Autodesk Inventor part; units mm, degrees
ref_plane "YZ Plane" through (0, 0, 0) normal (1, 0, 0) x (0, 1, 0)
ref_plane "XZ Plane" through (0, 0, 0) normal (0, 1, 0) x (-1, 0, 0)
ref_plane "XY Plane" through (0, 0, 0) normal (0, 0, 1) x (1, 0, 0)
sketch "Sketch1" plane through (0, 0, 0) normal (0, 1, 0) x (-1, 0, 0)
  line L0 (0.85, 10.55) -> (-0.85, 10.55)
  line L1 (-0.85, 10.55) -> (-0.85, -10.55)
  line L2 (-0.85, -10.55) -> (0.85, -10.55)
  line L3 (0.85, -10.55) -> (0.85, 10.55)
  line L4 (0.85, 10.55) -> (-0.85, -10.55) construction
  line L5 (-0.85, 10.55) -> (0.85, -10.55) construction
  line L6 (2.35, 12.05) -> (-2.35, 12.05)
  line L7 (-2.35, 12.05) -> (-2.35, -12.05)
  line L8 (-2.35, -12.05) -> (2.35, -12.05)
  line L9 (2.35, -12.05) -> (2.35, 12.05)
  point P0 (0, 0)
  dimension "d0" = 1.7
  dimension "d1" = 21.1
  dimension "d2" = 1.5
extrude "Extrusion1" add sketch "Sketch1" along normal blind 1.5
sketch "Sketch2" plane through (0, 0, 0) normal (0, -1, 0) x (1, 0, 0)
  line L0 (4.95, 12.05) -> (-6.05, 12.05)
  line L1 (-6.05, 12.05) -> (-6.05, -12.05)
  line L2 (-6.05, -12.05) -> (4.95, -12.05)
  line L3 (4.95, -12.05) -> (4.95, 12.05)
  line L4 (-2.35, 12.05) -> (2.35, 12.05)
  line L5 (-2.35, -12.05) -> (-2.35, 12.05)
  dimension "d5" = 11
  dimension "d6" = 3.7
extrude "Extrusion2" add sketch "Sketch2" along normal blind 2.4
sketch "Sketch3" plane through (0, 0, 0) normal (0, 1, 0) x (1, 0, 0)
  line L0 (-2.35, 12.05) -> (-2.35, -12.05)
  line L1 (-6.05, 12.05) -> (-2.35, 12.05)
  line L2 (-6.05, -12.05) -> (-6.05, 12.05)
  line L3 (-2.35, -12.05) -> (-6.05, -12.05)
  line L4 (2.35, -12.05) -> (2.35, 12.05)
  line L5 (4.95, -12.05) -> (2.35, -12.05)
  line L6 (4.95, 12.05) -> (4.95, -12.05)
  line L7 (2.35, 12.05) -> (4.95, 12.05)
  point P0 (0, 0)
extrude "Extrusion3" cut sketch "Sketch3" against normal blind 1.4
move faces "Move1" translate (0, 0, -1.5) faces at (0.7833, 0.5333, 12.05)
sketch "Sketch4" plane through (0, -2.4, 0) normal (0, -1, 0) x (1, 0, 0)
  line L0 (-0.85, -10.55) -> (0.85, -10.55)
  line L1 (-6.05, 10.55) -> (-6.05, -12.05)
  line L2 (2.35, -12.05) -> (4.95, -12.05)
  line L3 (-6.05, -10.55) -> (4.95, -10.55)
  line L4 (4.95, -10.55) -> (4.95, -12.05)
  line L5 (4.95, -12.05) -> (-6.05, -12.05)
  line L6 (-6.05, -12.05) -> (-6.05, -10.55)
  point P0 (0, 0)
extrude "Extrusion4" add sketch "Sketch4" along normal blind 1.8
move faces "Move2" translate (0, -1.4, 0) faces at (-0.2833, 0, 3.5167)
move faces "Move3" translate (0.5, 0, 0) faces at (-6.05, -1.7333, -4.0167)
move faces "Move4" translate (-0.5, 0, 0) faces at (4.95, -1.7333, -4.0167)
move faces "Move5" translate (0, 0, 1) faces at (-0.65, -2.0667, 10.55)
sketch "Sketch5" plane through (-5.55, -2.4, 11.55) normal (0, 0, 1) x (1, 0, 0)
  line L0 (4.7, 1) -> (4.7, 3.9)
  line L1 (3.2, 3.9) -> (4.7, 3.9)
  line L2 (3.2, 1) -> (3.2, 3.9)
  line L3 (3.2, 1) -> (0, 1)
  line L4 (0, 1) -> (0, 0)
  line L5 (10, 0) -> (0, 0)
  line L6 (10, 1) -> (10, 0)
  line L7 (10, 1) -> (7.9, 1)
  line L8 (7.9, 1) -> (7.9, 3.9)
  line L9 (6.4, 3.9) -> (7.9, 3.9)
  line L10 (6.4, 1) -> (6.4, 3.9)
  line L11 (6.4, 1) -> (4.7, 1)
  line L12 (4.7, 3.9) -> (6.4, 3.9)
  line L13 (4.7, 3.9) -> (6.4, 3.9)
  point P0 (5.55, 2.4)
extrude "Extrusion5" add sketch "Sketch5" along normal blind 1
move faces "Move6" translate (0, 0, -0.5) faces at (-0.2833, 0.5333, 11.55)
move faces "Move7" translate (0, 0.5, 0) faces at (-0.85, 0.5333, -3.35) (-0.2833, -1.4, -3.35)
sketch "Sketch6" plane through (2.35, -1.4, -12.05) normal (1, 0, 0) x (0, 0, -1)
  line L0 (-1.5, 2.9) -> (-23.1, 2.9)
  circle A0 centre (-3.41, 2.9) radius 0.75
  circle A1 centre (-5.95, 2.9) radius 0.75
  circle A2 centre (-8.49, 2.9) radius 0.75
  circle A3 centre (-11.03, 2.9) radius 0.75
  circle A4 centre (-13.57, 2.9) radius 0.75
  circle A5 centre (-16.11, 2.9) radius 0.75
  circle A6 centre (-18.65, 2.9) radius 0.75
  circle A7 centre (-21.19, 2.9) radius 0.75
  point P0 (-12.05, 1.4)
  dimension "d36" = 1.5
  dimension "d39" = 2.54
  dimension "d44" = 1.91
  dimension "d45" = 1.91
extrude "Extrusion6" cut sketch "Sketch6" against normal blind 2
equation "\"d44\" = d45"
properties part number "gyro_holder"
Could you check a few things on this model? Use its own coordinates, in mm. A direction names the side the tool comes from. Coordinates: 2 decimals unless noted, no trailing zeros. Order: outer loops, then holes, each group sorted by start corner. A loop starts at its lowest first (then second) coordinate and runs counter-clockwise, first axis right, second up. Notation, with made-up numbers: (-30, 30.5) - (27, 30.5) arc R17 cw to (27, 40.5) - close; hole circle Ø1 at (-29, 88.25). An arc over 180 degrees is marked (long way). Answer in a Markdown table with one row per item. Add a question column.
(1) On a 3-axis mill with a long thin cutter (end or side, diameter ignored), from which of +Z, -Z, +X, -X, +Y, -Y can I reach the whole of each face in a straight line? I mean faces 4 (the face through (1.61, 0.75, 6.62)), 5 (the face through (-0.85, 0, 0)), 6 (the face through (2.35, 0, 0)), 7 (the face through (2, 1.5, -2)). Say none if no direction works.
(2) If we mould it in two halves opening along X, with no side actions, what happens to faces 1 (the face through (-4, -1.4, 0)), 2 (the face through (-2.35, 0, 0)), 3 (the face through (0, 0, 11.05))? For each: released by +X, released by -X, zero draft, split by the parting line, or undercut.
(3) Will these pins go through, and if not, where does the flat tip stop? pin 1 (4 mm diameter, centred on x = -3.5, z = 3.5, fed in from -Y); pin 2 (1.9 mm diameter, centred on y = 0, z = -0.5, fed in from -X); pin 3 (2 mm diameter, centred on x = 0.5, y = -3, fed in from +Z); pin 4 (1.5 mm diameter, centred on y = 0.5, z = -1.5, fed in from +X).
(4) If we section it at B-B, the plane y = 0.25: Please give me the cut outline in (x, z), then the cut area to 3 significant figures.
(5) I need wall thicknesses on L1, parallel to X at y = -0.1, z = -2.5; L2, parallel to Y at x = -2.5, z = 0; L3, parallel to Y at x = 1, z = -5. Which ranges of each line are inside material? Lowest first, please.
(6) If we section it at A-A, the plane z = -8.64: Please give me the cut outline in (x, y).
(7) If we section it at D-D, the plane y = -2.7: Please give me the cut outline in (x, z), then the cut area to 3 significant figures.
(8) If we section it at C-C, the plane x = 2: Please give me the cut outline in (y, z).
Results are:
| question | item | result |
|---|---|---|
| 1 | face 4 | +X, +Y |
| 1 | face 5 | +Y |
| 1 | face 6 | +Z, -Z, +X, +Y |
| 1 | face 7 | +Z, -Z, +X, -X, +Y |
| 2 | face 1 | zero draft |
| 2 | face 2 | released by -X |
| 2 | face 3 | undercut |
| 3 | pin 1 | stops at y = -2.4 |
| 3 | pin 2 | stops at x = -2.35 |
| 3 | pin 3 | stops at z = 12.55 |
| 3 | pin 4 | stops at x = 2.35 |
| 4 | outline | (-2.35, -12.05) - (2.35, -12.05) - (2.35, 12.55) - (-2.35, 12.55) - close; hole (-0.85, -10.55) - (0.85, -10.55) - (0.85, 11.05) - (-0.85, 11.05) - close |
| 4 | area | 78.9 mm2 |
| 5 | L1 | x = -2.35 to -0.85, 0.85 to 2.35 |
| 5 | L2 | y = -2.4 to -1.4 |
| 5 | L3 | y = -2.4 to 1.5 |
| 6 | outline | (-5.55, -2.4) - (4.45, -2.4) - (4.45, -1.4) - (2.35, -1.4) - (2.35, 0.75) - (0.85, 0.75) - (0.85, -0.9) - (-0.85, -0.9) - (-0.85, 1.5) - (-2.35, 1.5) - (-2.35, -1.4) - (-5.55, -1.4) - close |
| 7 | outline | (-5.55, -12.05) - (4.45, -12.05) - (4.45, -10.55) - (-5.55, -10.55) - close |
| 7 | area | 15.0 mm2 |
| 8 | outline | (-4.2, -12.05) - (1.5, -12.05) - (1.5, -9.39) arc R0.75 cw to (1.5, -7.89) - (1.5, -6.85) arc R0.75 cw to (1.5, -5.35) - (1.5, -4.31) arc R0.75 cw to (1.5, -2.81) - (1.5, -1.77) arc R0.75 cw to (1.5, -0.27) - (1.5, 0.77) arc R0.75 cw to (1.5, 2.27) - (1.5, 3.31) arc R0.75 cw to (1.5, 4.81) - (1.5, 5.85) arc R0.75 cw to (1.5, 7.35) - (1.5, 8.39) arc R0.75 cw to (1.5, 9.89) - (1.5, 12.55) - (-2.4, 12.55) - (-2.4, -10.55) - (-4.2, -10.55) - close |
